```python
from build123d import *

# Parameters (mm, degrees)
F3_SIZE  = 0.49999
F1_W     = 1.9
F1_H     = 5
F1_H_2   = 6
F4_DEPTH = 3.45
F5_SIZE  = 0.99999
F6_R     = 1
F7_DEPTH = 6


# Not quite as in the source:
# - a fillet or chamfer is up to 0.001 mm smaller than in the source, because OpenCascade refuses the exact size


with BuildPart() as f2:
    # F0 (on Top) → F2 (revolve)
    with BuildSketch(Plane.XY):
        Polygon((0, -40.7), (0, 0), (-2.45, 0), (-2.45, -7.5), (-1.95, -7.5), (-1.95, -8.6), (-2.45, -8.6), (-2.45, -32.1), (-1.95, -32.1), (-1.95, -33.2), (-2.45, -33.2), (-2.45, -40.7), align=None)
    revolve(axis=Axis((0, -15.1539987261, 0), (0, -1, 0)))

    # F3 (size 0.5 in the source; OpenCascade refuses exactly that, so slightly less here)
    f3_edges = [f2.edges().sort_by_distance(p)[0] for p in [
        (2.45, -8.6, 0),
        (2.45, -33.2, 0),
        (2.45, -7.5, 0),
        (2.45, -32.1, 0),
    ]]
    chamfer(f3_edges, length=F3_SIZE)

    # F1 (on Top) → F4 (join)
    with BuildSketch(Plane.XY):
        with Locations((0, -4.5)):
            Rectangle(F1_W, F1_H)
        with Locations((0, -36.7)):
            Rectangle(F1_W, F1_H_2)
    extrude(amount=F4_DEPTH)

    # F5 (size 1 in the source; OpenCascade refuses exactly that, so slightly less here)
    f5_edges = [f2.edges().sort_by_distance(p)[0] for p in [
        (0, -33.7, 3.45),
        (0, -2, 3.45),
    ]]
    chamfer(f5_edges, length=F5_SIZE)

    # F6 (on face) → F7 (cut)
    with BuildSketch(Plane.XZ.offset(40.7)):
        Circle(F6_R)
    extrude(amount=-F7_DEPTH, mode=Mode.SUBTRACT)


solid = f2.part
```
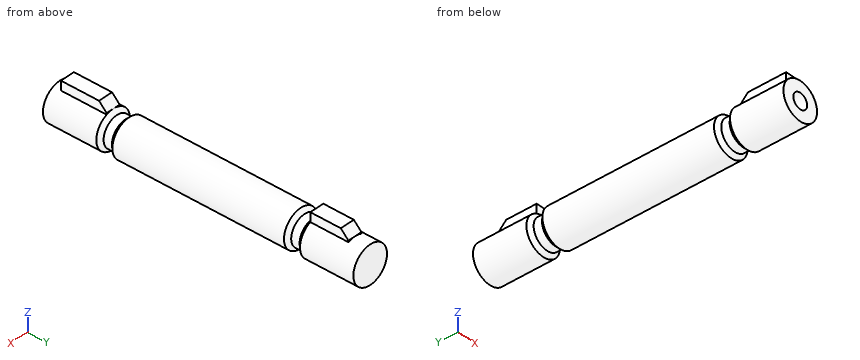
Input: part model. Units: mm. Frame: model coordinates. Give positions to 0.01 mm unless a question says otherwise; leave off trailing zeros. Loops run counter-clockwise (first coordinate to the right, second up) from the corner with the lowest first, then second, coordinate; pieces in that order, holes last. Notation, with made-up numbers: (1, 52.5) -> (56, 52.5) arc R19 cw to (56, 60.5) -> close; hole circle Ø4 at (36, 22.5). An arc over 180 degrees is marked (long way). Use a Markdown table: item, result.
Q1. Section query A-A, the plane z = 3. Return the cut outline in (x, y), plus the area to 3 significant figures.
Entries:
| item | result |
|---|---|
| outline | (-0.95, -39.7) -> (0.95, -39.7) -> (0.95, -34.25) -> (-0.95, -34.25) -> close; (-0.95, -7) -> (0.95, -7) -> (0.95, -2.55) -> (-0.95, -2.55) -> close |
| area | 18.8 mm² |
Q2. Section query B-B, the plane y = -4. Return the cut outline in (x, z).
Entries:
| item | result |
|---|---|
| outline | (-0.95, 2.26) arc R2.45 ccw (long way) to (0.95, 2.26) -> (0.95, 3.45) -> (-0.95, 3.45) -> close |
Q3. Section query D-D, the plane y = -15. Return the cut outline in (x, z), plus the area to 3 significant figures.
Entries:
| item | result |
|---|---|
| outline | circle Ø4.9 at (0, 0) |
| area | 18.9 mm² |
Q4. First-contact query: P1, Ø0.6, axis at y = -5.5, z = 3, coming from the +X side; P2, Ø2, axis at x = 0.5, z = 1.5, coming from the +Y side; P3, Ø0.6, axis at y = -37, z = 2.5, coming from the +X side; P4, Ø0.6, axis at y = -5.5, z = 2.5, coming from the -X side. Flat tips, straight axial feed; report the tip coordinate or a pass-through.
Entries:
| item | result |
|---|---|
| P1 | stops at x = 0.95 |
| P2 | stops at y = 0 |
| P3 | stops at x = 1.08 |
| P4 | stops at x = -1.08 |
Q5. Ray query, probe 1 along Z at (x, y) = (0, -38.15); probe 2 along Y at (x, z) = (-1.15, 1.95); probe 3 along Y at (x, z) = (-0.95, 1.9). Return the intervals inside material, ascending. Write a range as from..to.
Entries:
| item | result |
|---|---|
| probe 1 | z = -2.45..-1, 1..3.45 |
| probe 2 | y = -40.7..-33.51, -31.79..-8.91, -7.19..0 |
| probe 3 | y = -40.7..-33.37, -31.93..-8.77, -7.33..0 |
